For this review, take the finished solid that the model builds, in its own axes (mm). A direction names the side the tool comes from. Round coordinates to 2 decimals unless told otherwise and drop trailing zeros. Order: outer loops, then holes, each group sorted by start corner. A loop starts at its lowest first (then second) coordinate and runs counter-clockwise, first axis right, second up. Notation, with made-up numbers: (84, 60.25) - (133, 60.25) arc R11 ccw to (133, 73.25) - close; hole circle Ø10 at (19.5, -38.75). An arc over 180 degrees is marked (long way). One line per item, written item: value.
Autodesk Inventor part; units mm, degrees
ref_plane "YZ Plane" through (0, 0, 0) normal (1, 0, 0) x (0, 1, 0)
ref_plane "XZ Plane" through (0, 0, 0) normal (0, 1, 0) x (-1, 0, 0)
ref_plane "XY Plane" through (0, 0, 0) normal (0, 0, 1) x (1, 0, 0)
sketch "Sketch1" plane through (0, 0, 0) normal (0, 0, 1) x (1, 0, 0)
  line L0 (0, 0) -> (25.4, 0)
  line L1 (0, 0) -> (0, 11.43)
  line L2 (3.175, 11.43) -> (3.175, 3.175)
  line L3 (3.175, 3.175) -> (25.4, 3.175)
  line L4 (0, 11.43) -> (3.175, 11.43)
  line L5 (25.4, 3.175) -> (25.4, 0)
  dimension "d0" = 25.4
  dimension "d2" = 11.43
  dimension "d3" = 90
  dimension "d4" = 3.175
extrude "Extrusion1" add sketch "Sketch1" along normal blind 200.025
sketch "Sketch2" plane through (0, -3.175, 203.2) normal (0, 0, 1) x (1, 0, 0)
  line L0 (25.4, 0) -> (0, 0)
  line L1 (0, 0) -> (0, -19.05)
  line L2 (0, -19.05) -> (25.4, -19.05)
  line L3 (25.4, -19.05) -> (25.4, 0)
edge flange "Flange1" height 25.4 angle 90 thickness 3.175 bend radius 3.175 thickness toward (0, 0, 1) relief straight relief width 3.175 relief depth 1.5875 edges at (12.7, 0, 200.025) wall of the first edge with corners at (25.4, -3.175, 203.2) (0, -3.175, 203.2) (0, -22.225, 203.2) (25.4, -22.225, 203.2)
bend "Bend1"
corner "Corner1"
equation "\"d7\" = BendReliefWidth"
equation "\"d8\" = BendReliefDepth"
equation "\"d9\" = MinimumRemnant"
equation "\"d10\" = BendRadius"
equation "\"d13\" = BendRadius"
equation "\"d14\" = CornerReliefSize"
equation "\"d15\" = GapSize"
equation "\"d16\" = JacobiRadiusSize"
equation "\"BendRadius\" = Thickness"
equation "\"BendReliefWidth\" = Thickness"
equation "\"BendReliefDepth\" = 0.5 * Thickness"
equation "\"CornerReliefSize\" = 4 * Thickness"
equation "\"MinimumRemnant\" = 2 * Thickness"
equation "\"TransitionRadius\" = BendRadius"
equation "\"JacobiRadiusSize\" = Thickness"
equation "\"GapSize\" = Thickness"
properties part number "Bent L"
Item 1: For P1, Ø12, axis at x = 22.5, z = 127.5, coming from the +Y side (3 decimals); P2, Ø1.5, axis at x = 17.5, y = 2, coming from the +Z side; P3, Ø12, axis at x = 15.5, y = -1, coming from the +Z side (3 decimals); P4, Ø4, axis at y = 8.5, z = 64.5, coming from the +X side (3 decimals), all flat-tipped, find the tip position at first contact; note any pin that passes through.
Returned:
P1: y = 3.175
P2: z = 204.58
P3: z = 206.375
P4: x = 3.175
Item 2: Take a section at C-C (y = -9). Write out the cut boundary in (x, z) (3 decimals), plus the area to 3 significant figures.
Returned:
outline: (0, 203.2) - (25.4, 203.2) - (25.4, 206.375) - (0, 206.375) - close
area: 80.6 mm^2
Item 3: Take a section at D-D (y = 9.5). Write out the cut boundary in (x, z) (3 decimals), plus the area to 3 significant figures.
Returned:
outline: (0, 0) - (3.175, 0) - (3.175, 200.025) - (0, 200.025) - close
area: 635 mm^2
Item 4: Take a section at B-B (z = 106.5). Write out the cut boundary in (x, y) (3 decimals).
Returned:
outline: (0, 0) - (25.4, 0) - (25.4, 3.175) - (3.175, 3.175) - (3.175, 11.43) - (0, 11.43) - close
Item 5: Machinability: for faces 1 (the flat face through (14, 3.175, 99)), 2 (the flat face through (13, -13, 203.2)), 3 (the flat face through (2, 7, 200.025)), which of the approach directions +Z, -Z, +X, -X, +Y, -Y give a long, thin tool a straight path to every point of the face, cutting with its end or side? Answer none if there is none.
Returned:
face 1: +Z, -Z, +X, +Y
face 2: -Z, +X, -X, -Y
face 3: +Z, +X, -X, +Y
Item 6: Wall thickness on line 1 (Z direction, x = 2, y = 3.5) (3 decimals); line 2 (Y direction, x = 24.75, z = 118) (3 decimals): over which ranges is each line inside the solid? List them lowest first.
Returned:
line 1: 0 to 200.025
line 2: 0 to 3.175
Item 7: Take a section at A-A (x = 18.25). Write out the cut boundary in (y, z) (3 decimals).
Returned:
outline: (-22.225, 203.2) - (-3.175, 203.2) arc R3.175 cw to (0, 200.025) - (0, 0) - (3.175, 0) - (3.175, 200.025) arc R6.35 ccw to (-3.175, 206.375) - (-22.225, 206.375) - close
